from build123d import *

# Parameters (mm, degrees)
SKETCH1_R           = 2
SKETCH1_R_2         = 1.5
SKETCH1_W           = 3
SKETCH1_H           = 5
SKETCH1_R_3         = 5
SKETCH1_H_2         = 7
BOSS_EXTRUDE1_DEPTH = 3


with BuildPart() as part:
    # Sketch1 → Boss-Extrude1 (new body)
    with BuildSketch(Plane(origin=(0, 0, 0), x_dir=(1, 0, 0), z_dir=(0, 1, 0))):
        with BuildLine():
            ThreePointArc((10.699698215, 29.641238244), (11.406804996, 29.934131463), (11.699698215, 30.641238244))
            Line((11.699698215, 30.641238244), (11.699698215, 38.128019164))
            Line((11.699698215, 38.128019164), (11.699698215, 45.611855364))
            ThreePointArc((11.699698215, 45.611855364), (7.306299933, 56.218457082), (-3.300301785, 60.611855364))
            Line((-3.300301785, 60.611855364), (-86.492412558, 60.611855364))
            ThreePointArc((-86.492412558, 60.611855364), (-97.099014275, 56.218457082), (-101.492412558, 45.611855364))
            Line((-101.492412558, 45.611855364), (-101.492412558, 38.128019164))
            Line((-101.492412558, 38.128019164), (-101.492412558, 29.641238244))
            Line((-101.492412558, 29.641238244), (-98.492412558, 29.641238244))
            Line((-98.492412558, 29.641238244), (-98.492412558, 22.141238244))
            Line((-98.492412558, 22.141238244), (-95.492412558, 22.141238244))
            Line((-95.492412558, 22.141238244), (-95.492412558, 7.141238244))
            Line((-95.492412558, 7.141238244), (-98.492412558, 7.141238244))
            Line((-98.492412558, 7.141238244), (-98.492412558, -22.858761756))
            Line((-98.492412558, -22.858761756), (-95.492412558, -22.858761756))
            Line((-95.492412558, -22.858761756), (-95.492412558, -37.858761756))
            Line((-95.492412558, -37.858761756), (-98.492412558, -37.858761756))
            Line((-98.492412558, -37.858761756), (-98.492412558, -40.358761756))
            Line((-98.492412558, -40.358761756), (-100.492412558, -40.358761756))
            ThreePointArc((-100.492412558, -40.358761756), (-101.199519339, -40.651654975), (-101.492412558, -41.358761756))
            Line((-101.492412558, -41.358761756), (-101.492412558, -46.358761756))
            ThreePointArc((-101.492412558, -46.358761756), (-101.785305776, -47.065868537), (-102.492412558, -47.358761756))
            Line((-102.492412558, -47.358761756), (-124.579684665, -47.358761756))
            ThreePointArc((-124.579684665, -47.358761756), (-128.115218571, -48.82322785), (-129.579684665, -52.358761756))
            Line((-129.579684665, -52.358761756), (-129.579684665, -79.388144636))
            ThreePointArc((-129.579684665, -79.388144636), (-120.7928881, -100.601348072), (-99.579684665, -109.388144636))
            Line((-99.579684665, -109.388144636), (9.786970322, -109.388144636))
            ThreePointArc((9.786970322, -109.388144636), (31.000173758, -100.601348072), (39.786970322, -79.388144636))
            Line((39.786970322, -79.388144636), (39.786970322, -52.358761756))
            ThreePointArc((39.786970322, -52.358761756), (38.322504228, -48.82322785), (34.786970322, -47.358761756))
            Line((34.786970322, -47.358761756), (12.699698215, -47.358761756))
            ThreePointArc((12.699698215, -47.358761756), (11.992591434, -47.065868537), (11.699698215, -46.358761756))
            Line((11.699698215, -46.358761756), (11.699698215, -41.358761756))
            ThreePointArc((11.699698215, -41.358761756), (11.406804997, -40.651654975), (10.699698215, -40.358761756))
            Line((10.699698215, -40.358761756), (8.699698215, -40.358761756))
            Line((8.699698215, -40.358761756), (8.699698215, -37.858761756))
            Line((8.699698215, -37.858761756), (5.699698215, -37.858761756))
            Line((5.699698215, -37.858761756), (5.699698215, -22.858761756))
            Line((5.699698215, -22.858761756), (8.699698215, -22.858761756))
            Line((8.699698215, -22.858761756), (8.699698215, 7.141238244))
            Line((8.699698215, 7.141238244), (5.699698215, 7.141238244))
            Line((5.699698215, 7.141238244), (5.699698215, 22.141238244))
            Line((5.699698215, 22.141238244), (8.699698215, 22.141238244))
            Line((8.699698215, 22.141238244), (8.699698215, 29.641238244))
            Line((8.699698215, 29.641238244), (10.699698215, 29.641238244))
        make_face()
        with Locations(Location((-64.542412558, -87.858761756, 0), (0, 0, 270))):
            Circle(SKETCH1_R, mode=Mode.SUBTRACT)
        with Locations(Location((-91.992412558, -45.858761756, 0), (0, 0, 270))):
            Circle(SKETCH1_R_2, mode=Mode.SUBTRACT)
        with Locations((-96.992412558, -44.858761756)):
            Rectangle(SKETCH1_W, SKETCH1_H, mode=Mode.SUBTRACT)
        with Locations(Location((-44.896357171, -91.07147213, 0), (0, 0, 270))):
            Circle(SKETCH1_R_3, mode=Mode.SUBTRACT)
        with Locations(Location((-24.942412558, -87.858761756, 0), (0, 0, 270))):
            Circle(SKETCH1_R, mode=Mode.SUBTRACT)
        with Locations(Location((2.199698215, -45.858761756, 0), (0, 0, 270))):
            Circle(SKETCH1_R_2, mode=Mode.SUBTRACT)
        with Locations((7.199698215, -44.858761756)):
            Rectangle(SKETCH1_W, SKETCH1_H, mode=Mode.SUBTRACT)
        with BuildLine():
            Line((-52.896357171, 5.611855364), (-56.896357171, 5.611855364))
            ThreePointArc((-56.896357171, 5.611855364), (-59.017677515, 6.49053502), (-59.896357171, 8.611855364))
            Line((-59.896357171, 8.611855364), (-59.896357171, 23.611855364))
            ThreePointArc((-59.896357171, 23.611855364), (-59.017677515, 25.733175707), (-56.896357171, 26.611855364))
            Line((-56.896357171, 26.611855364), (-52.896357171, 26.611855364))
            ThreePointArc((-52.896357171, 26.611855364), (-50.775036828, 25.733175707), (-49.896357171, 23.611855364))
            Line((-49.896357171, 23.611855364), (-49.896357171, 8.611855364))
            ThreePointArc((-49.896357171, 8.611855364), (-50.775036828, 6.49053502), (-52.896357171, 5.611855364))
        make_face(mode=Mode.SUBTRACT)
        with Locations(Location((-91.992412558, 30.187503495, 0), (0, 0, 270))):
            Circle(SKETCH1_R_2, mode=Mode.SUBTRACT)
        with Locations((-96.992412558, 35.141238244)):
            Rectangle(SKETCH1_W, SKETCH1_H_2, mode=Mode.SUBTRACT)
        with Locations(Location((-67.492412558, 24.11185536, 0), (0, 0, 270))):
            Circle(SKETCH1_R_2, mode=Mode.SUBTRACT)
        with BuildLine():
            Line((-78.392412558, 39.891238244), (-91.592412558, 39.891238244))
            ThreePointArc((-91.592412558, 39.891238244), (-92.935915442, 40.44773536), (-93.492412558, 41.791238244))
            Line((-93.492412558, 41.791238244), (-93.492412558, 41.991238244))
            ThreePointArc((-93.492412558, 41.991238244), (-92.935915442, 43.334741128), (-91.592412558, 43.891238244))
            Line((-91.592412558, 43.891238244), (-78.392412558, 43.891238244))
            ThreePointArc((-78.392412558, 43.891238244), (-77.048909673, 43.334741128), (-76.492412558, 41.991238244))
            Line((-76.492412558, 41.991238244), (-76.492412558, 41.791238244))
            ThreePointArc((-76.492412558, 41.791238244), (-77.048909673, 40.44773536), (-78.392412558, 39.891238244))
        make_face(mode=Mode.SUBTRACT)
        with Locations(Location((-44.896357171, -6.07147213, 0), (0, 0, 270))):
            Circle(SKETCH1_R_3, mode=Mode.SUBTRACT)
        with BuildLine():
            ThreePointArc((-32.896357171, 26.611855364), (-30.775036828, 25.733175707), (-29.896357171, 23.611855364))
            Line((-29.896357171, 23.611855364), (-29.896357171, 8.611855364))
            ThreePointArc((-29.896357171, 8.611855364), (-30.775036828, 6.49053502), (-32.896357171, 5.611855364))
            Line((-32.896357171, 5.611855364), (-36.896357171, 5.611855364))
            ThreePointArc((-36.896357171, 5.611855364), (-39.017677515, 6.49053502), (-39.896357171, 8.611855364))
            Line((-39.896357171, 8.611855364), (-39.896357171, 23.611855364))
            ThreePointArc((-39.896357171, 23.611855364), (-39.017677515, 25.733175707), (-36.896357171, 26.611855364))
            Line((-36.896357171, 26.611855364), (-32.896357171, 26.611855364))
        make_face(mode=Mode.SUBTRACT)
        with Locations(Location((-22.300301785, 24.11185536, 0), (0, 0, 270))):
            Circle(SKETCH1_R_2, mode=Mode.SUBTRACT)
        with Locations(Location((-44.896357171, 43.611855364, 0), (0, 0, 270))):
            Circle(SKETCH1_R, mode=Mode.SUBTRACT)
        with BuildLine():
            Line((3.699698215, 41.991238244), (3.699698215, 41.791238244))
            ThreePointArc((3.699698215, 41.791238244), (3.143201099, 40.44773536), (1.799698215, 39.891238244))
            Line((1.799698215, 39.891238244), (-11.400301785, 39.891238244))
            ThreePointArc((-11.400301785, 39.891238244), (-12.743804669, 40.44773536), (-13.300301785, 41.791238244))
            Line((-13.300301785, 41.791238244), (-13.300301785, 41.991238244))
            ThreePointArc((-13.300301785, 41.991238244), (-12.743804669, 43.334741128), (-11.400301785, 43.891238244))
            Line((-11.400301785, 43.891238244), (1.799698215, 43.891238244))
            ThreePointArc((1.799698215, 43.891238244), (3.143201099, 43.334741128), (3.699698215, 41.991238244))
        make_face(mode=Mode.SUBTRACT)
        with Locations(Location((2.199698215, 30.187503495, 0), (0, 0, 270))):
            Circle(SKETCH1_R_2, mode=Mode.SUBTRACT)
        with Locations((7.199698215, 35.141238244)):
            Rectangle(SKETCH1_W, SKETCH1_H_2, mode=Mode.SUBTRACT)
    extrude(amount=BOSS_EXTRUDE1_DEPTH)


solid = part.part
For this review, take the finished solid that the model builds, in its own axes (mm). Coordinates: 2 decimals unless noted, no trailing zeros. Loops run counter-clockwise (first coordinate to the right, second up) from the corner with the lowest first, then second, coordinate; pieces in that order, holes last. Notation, with made-up numbers: (87.25, 43.25) - (140.25, 43.25) arc R24 ccw to (140.25, 73.25) - close; hole circle Ø8 at (-30, -22.5). An arc over 180 degrees is marked (long way). Use a Markdown table: item, result. Add a question column.
Item 1: We need section C-C (z = 19). Give the boundary of the cut face in (x, y).
Item 2: We need section A-A (z = -34.5). Give the boundary of the cut face in (x, y).
Item 3: We need section B-B (z = -13). Give the boundary of the cut face in (x, y).
Item 4: For line 1 (X direction, y = 0.3, z = -30.5); line 2 (X direction, y = 2.65, z = -37); line 3 (Z direction, x = -52.5, y = 0.3), list the stretches that pass through material, from the lowest coordinate up.
Item 5: We need section D-D (y = 2.45). Give the number of separate pieces and of enclosed holes in the cut face, and give its area (3 significant figures).
Item 6: Insertion check: pin 1 Ø1.5 at (y, z) = (1, -15) entering from +X; pin 2 Ø1.5 at (x, y) = (-97.5, 1) entering from -Z; pin 3 Ø0.9 at (y, z) = (1.5, 44) entering from -X. Each pin has a flat end and moves straight along its axis. Give the tip position at first contact, or say it passes through.
Item 7: Mouldability with a two-part tool opening along X and no side actions: class faces 1 (the face through (-96.982, 1.479, -56.334)), 2 (the face through (30.8, 1.5, 100.8)), 3 (the face through (-63.191, 1.479, 86.385)) as pulls with the +X half, pulls with the -X half, needs draft (parallel to the pull), parting line crosses it, or undercut.
Results list:
| question | item | result |
|---|---|---|
| 1 | outline | (-98.49, 0) - (8.7, 0) - (8.7, 3) - (-98.49, 3) - close |
| 2 | outline | (-101.49, 0) - (-98.49, 0) - (-98.49, 3) - (-101.49, 3) - close; (-95.49, 0) - (5.7, 0) - (5.7, 3) - (-95.49, 3) - close; (8.7, 0) - (11.7, 0) - (11.7, 3) - (8.7, 3) - close |
| 3 | outline | (-95.49, 0) - (-59.9, 0) - (-59.9, 3) - (-95.49, 3) - close; (-49.9, 0) - (-39.9, 0) - (-39.9, 3) - (-49.9, 3) - close; (-29.9, 0) - (5.7, 0) - (5.7, 3) - (-29.9, 3) - close |
| 4 | line 1 | x = -101.49 to -93.46, -90.53 to 0.73, 3.67 to 11.69 |
| 4 | line 2 | x = -101.49 to -98.49, -95.49 to 5.7, 8.7 to 11.7 |
| 4 | line 3 | z = -60.61 to -26.59, -5.64 to 109.39 |
| 5 | separate pieces | 1 |
| 5 | enclosed holes | 19 |
| 5 | area | 20,800 mm^2 |
| 6 | pin 1 | stops at x = 5.7 |
| 6 | pin 2 | stops at z = -56.56 |
| 6 | pin 3 | stops at x = -101.49 |
| 7 | face 1 | pulls with the -X half |
| 7 | face 2 | pulls with the +X half |
| 7 | face 3 | undercut |
